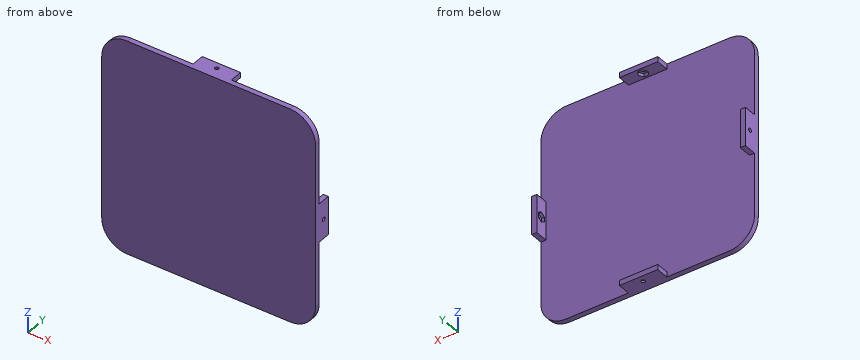
```python
from build123d import *

# Parameters (mm, degrees)
ESQUISSE1_W                  = 212.09
ESQUISSE1_H                  = 212.09
BOSS_EXTRU_1_DEPTH           = 5.08
ESQUISSE2_W                  = 38.1
ESQUISSE2_H                  = 5.08
ESQUISSE2_W_2                = 5.08
ESQUISSE2_H_2                = 38.1
BOSS_EXTRU_2_DEPTH           = 12.7
CONG_1_R                     = 25.4
D_GAGEMENT_61_D              = 3.7973
ENL_V_MAT_EXTRU_1_DEPTH      = 3
R_P_TITION_CIRCULAIRE1_COUNT = 4


with BuildPart() as part:
    # Esquisse1 → Boss.-Extru.1 (new body)
    with BuildSketch(Plane(origin=(0, 0, 0), x_dir=(1, 0, 0), z_dir=(0, 1, 0))):
        Rectangle(ESQUISSE1_W, ESQUISSE1_H)
    extrude(amount=BOSS_EXTRU_1_DEPTH)

    # Esquisse2 → Boss.-Extru.2 (add)
    with BuildSketch(Plane(origin=(0, 5.08, 0), x_dir=(1, 0, 0), z_dir=(0, 1, 0))):
        with Locations((0, -103.505)):
            Rectangle(ESQUISSE2_W, ESQUISSE2_H)
        with Locations((-103.505, 0)):
            Rectangle(ESQUISSE2_W_2, ESQUISSE2_H_2)
        with Locations((0, 103.505)):
            Rectangle(ESQUISSE2_W, ESQUISSE2_H)
        with Locations((103.505, 0)):
            Rectangle(ESQUISSE2_W_2, ESQUISSE2_H_2)
    extrude(amount=BOSS_EXTRU_2_DEPTH)

    # Congé1
    cong_1_edges = [part.edges().sort_by_distance(p)[0] for p in [
        (-106.045, 2.54, -106.045),
        (106.045, 2.54, -106.045),
        (106.045, 2.54, 106.045),
        (-106.045, 2.54, 106.045),
    ]]
    fillet(cong_1_edges, radius=CONG_1_R)

    # Dégagement #61 (through all)
    with Locations(Plane.XY.offset(106.045)):
        with Locations((0, 11.43)):
            d_gagement_61 = Hole(D_GAGEMENT_61_D / 2)

    # Esquisse5 → Enlèv. mat.-Extru.1 (cut)
    with BuildSketch(Plane.XY.offset(-100.965)):
        Polygon((2.453738644, 15.68), (-2.453738644, 15.68), (-4.907477288, 11.43), (-2.453738644, 7.18), (2.453738644, 7.18), (4.907477288, 11.43), align=None)
    enl_v_mat_extru_1 = extrude(amount=-ENL_V_MAT_EXTRU_1_DEPTH, mode=Mode.SUBTRACT)

    # Répétition circulaire1: Dégagement #61, Enlèv. mat.-Extru.1 ×4 about axis
    r_p_tition_circulaire1_axis = Axis((0, 0, 0), (0, 1, 0))
    add([d_gagement_61.rotate(r_p_tition_circulaire1_axis, i * 360 / R_P_TITION_CIRCULAIRE1_COUNT) for i in range(1, R_P_TITION_CIRCULAIRE1_COUNT)], mode=Mode.SUBTRACT)
    add([enl_v_mat_extru_1.rotate(r_p_tition_circulaire1_axis, i * 360 / R_P_TITION_CIRCULAIRE1_COUNT) for i in range(1, R_P_TITION_CIRCULAIRE1_COUNT)], mode=Mode.SUBTRACT)


solid = part.part
```
Design review of the part built by this model. Coordinates are the model's own, in mm. Round coordinates to 2 decimals unless told otherwise and drop trailing zeros. Write each loop counter-clockwise with the first axis right and the second up, starting at its lowest first coordinate (ties: lowest second). Pieces come first, ordered by that corner, then holes.
Item 1: We need section A-A on x = -16.5. Write out the cut boundary in (y, z) (3 decimals).
Item 2: Clearance check with flat-ended pins moving along their axes: pin 1 Ø3 at (x, z) = (80, -10.5) entering from +Y; pin 2 Ø5.5 at (y, z) = (9.5, -104.5) entering from -X; pin 3 Ø4 at (x, y) = (-103, 13) entering from +Z. State where each tip first meets the part, or that it passes through.
Item 3: For probe 1 along Y at (x, z) = (105, 0); probe 2 along Z at (x, y) = (13, 11.25) (3 decimals); probe 3 along Y at (x, z) = (-83.5, -66), list the stretches that pass through material, from the lowest coordinate up.
Item 4: We need section C-C on x = 43. Write out the cut boundary in (y, z) (3 decimals).
Item 5: We need section B-B on z = -72. Write out the cut boundary in (x, y) (3 decimals), and give its area (3 significant figures).
Returned:
1. outline: (0, -106.045) - (17.78, -106.045) - (17.78, -100.965) - (5.08, -100.965) - (5.08, 100.965) - (17.78, 100.965) - (17.78, 106.045) - (0, 106.045) - close
2. pin 1: stops at y = 5.08
2. pin 2: stops at x = -19.05
2. pin 3: stops at z = 19.05
3. probe 1: y = 0 to 9.53, 13.33 to 17.78
3. probe 2: z = -106.045 to -100.965, 100.965 to 106.045
3. probe 3: y = 0 to 5.08
4. outline: (0, -106.045) - (5.08, -106.045) - (5.08, 106.045) - (0, 106.045) - close
5. outline: (-106.045, 0) - (106.045, 0) - (106.045, 5.08) - (-106.045, 5.08) - close
5. area: 1,080 mm2
